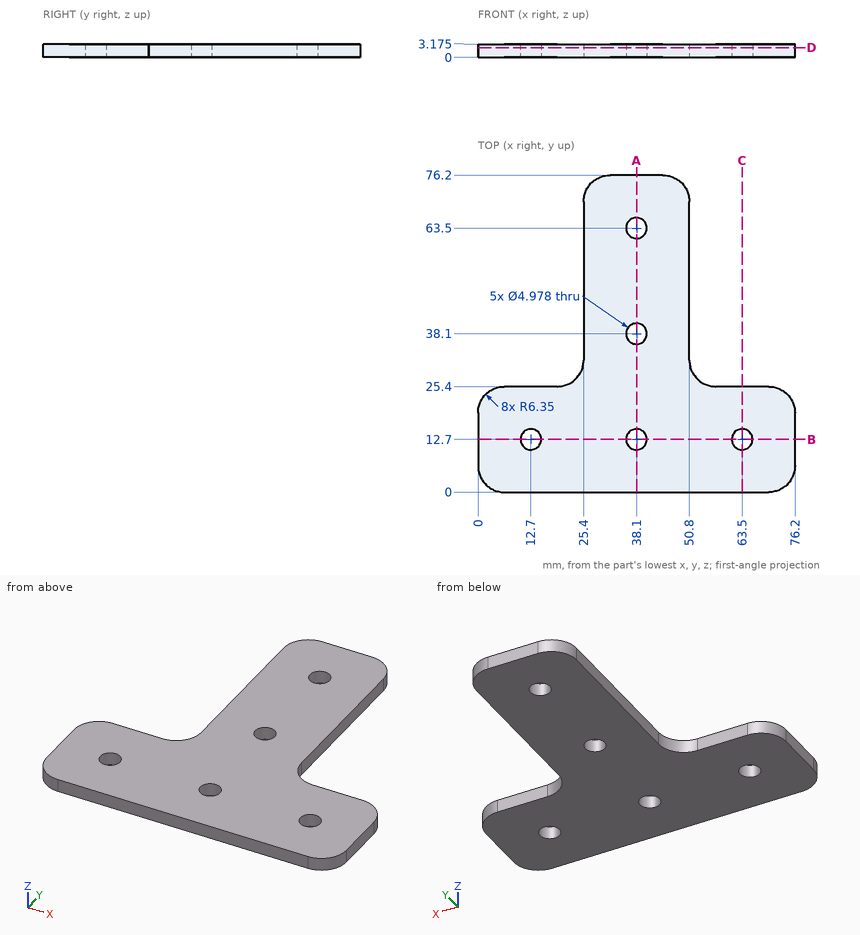
Study the drawing (mm; zero at the part's minimum x, y, z) and answer. Give positions to 0.01 mm unless a question says otherwise; leave off trailing zeros. Order: outer loops, then holes, each group sorted by start corner. A loop starts at its lowest first (then second) coordinate and runs counter-clockwise, first axis right, second up. Notation, with made-up numbers: (-6.75, 62.5) - (44.25, 62.5) arc R24 ccw to (44.25, 82.5) - close; hole circle Ø4 at (35.5, 14.25). An arc over 180 degrees is marked (long way). Use one line per item in the form item = value. Start each with the question number.
(1) Consider line 1 (Y direction, x = 38.1, z = 2.4); line 2 (Y direction, x = 40, z = 2.25); line 3 (Y direction, x = 31.5, z = 2.65) (1 decimal). Determine where each line is inside the solid, lowest interval first. Write a range as from..to.
(2) A cutting plane is placed at C-C, the plane x = 63.5. Write down the section's boundary in (y, z) (1 decimal).
(3) A cutting plane is placed at D-D, the plane z = 2.3. Write down the section's boundary in (x, y).
(4) Flat-ended cylindrical pins translate along their axes: pin 1 Ø1.6 at (x, z) = (62.5, 1.5) entering from +Y; pin 2 Ø1 at (y, z) = (44, 1) entering from +X. Find the tip coordinate at first contact, or state that the pin passes through.
(5) A cutting plane is placed at A-A, the plane x = 38.1. Write down the section's boundary in (y, z) (1 decimal).
Ans:
q1.line_1 = 0..10.21, 15.19..35.61, 40.59..61.01, 65.99..76.2
q1.line_2 = 0..11.09, 14.31..36.49, 39.71..61.89, 65.11..76.2
q1.line_3 = 0..76.2
q2.outline = (0, 0) - (10.2, 0) - (10.2, 3.2) - (0, 3.2) - close; (15.2, 0) - (25.4, 0) - (25.4, 3.2) - (15.2, 3.2) - close
q3.outline = (0, 6.35) arc R6.35 ccw to (6.35, 0) - (69.85, 0) arc R6.35 ccw to (76.2, 6.35) - (76.2, 19.05) arc R6.35 ccw to (69.85, 25.4) - (57.15, 25.4) arc R6.35 cw to (50.8, 31.75) - (50.8, 69.85) arc R6.35 ccw to (44.45, 76.2) - (31.75, 76.2) arc R6.35 ccw to (25.4, 69.85) - (25.4, 31.75) arc R6.35 cw to (19.05, 25.4) - (6.35, 25.4) arc R6.35 ccw to (0, 19.05) - close; hole circle Ø4.98 at (12.7, 12.7); hole circle Ø4.98 at (38.1, 12.7); hole circle Ø4.98 at (38.1, 38.1); hole circle Ø4.98 at (38.1, 63.5); hole circle Ø4.98 at (63.5, 12.7)
q4.pin_1 = 25.4
q4.pin_2 = 50.8
q5.outline = (0, 0) - (10.2, 0) - (10.2, 3.2) - (0, 3.2) - close; (15.2, 0) - (35.6, 0) - (35.6, 3.2) - (15.2, 3.2) - close; (40.6, 0) - (61, 0) - (61, 3.2) - (40.6, 3.2) - close; (66, 0) - (76.2, 0) - (76.2, 3.2) - (66, 3.2) - close
